Input: part model. Units: mm. Frame: model coordinates. Face numbers are marked on the shaded views. A direction names the side the tool comes from. Give positions to 0.01 mm unless a question says otherwise; leave off trailing zeros. Loops run counter-clockwise (first coordinate to the right, second up) from the corner with the lowest first, then second, coordinate; pieces in that order, holes last. Notation, with made-up numbers: (56.5, 53.25) -> (97.5, 53.25) arc R22 cw to (97.5, 85.25) -> close; hole circle Ø3 at (49.5, -38). An arc over 180 degrees is marked (long way). Answer in a Markdown table with one row per item. Add a question column.
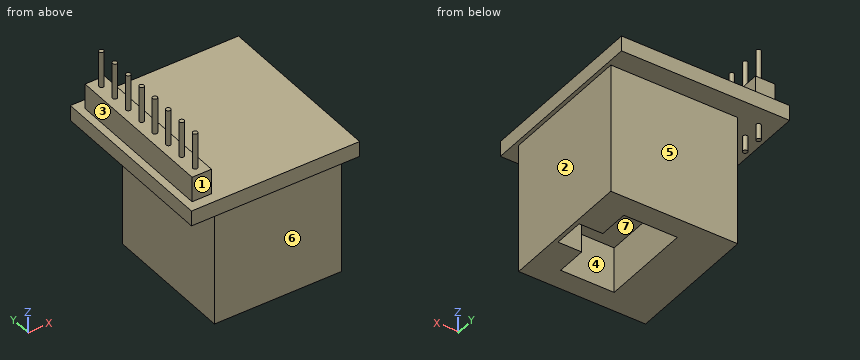
```python
from build123d import *

# Parameters (mm, degrees)
F0_W          = 16.6
F0_H          = 17.5
F1_DEPTH      = 17
F3_DEPTH      = 6
F4_W          = 22
F4_H          = 23
F4_W_2        = 16.6
F4_H_2        = 17.5
F5_DEPTH      = 2
F6_W          = 2.54
F6_H          = 2.54
F6_R          = 0.3
F7_DEPTH      = 3.3
F8_DEPTH      = 8
F8_DEPTH_BACK = 4


with BuildPart() as f1:
    # F0 (on Top) → F1 (new body)
    with BuildSketch(Plane.XY):
        Rectangle(F0_W, F0_H)
    extrude(amount=F1_DEPTH)

    # F2 (on face) → F3 (cut)
    with BuildSketch(Plane(origin=(0, 0, 0), x_dir=(1, 0, 0), z_dir=(0, 0, -1))):
        Polygon((7.8, -2), (7.8, 0), (7.8, 2), (4.7, 2), (4.7, 6), (-2.3, 6), (-2.3, 0), (-2.3, -6), (4.7, -6), (4.7, -2), align=None)
    extrude(amount=-F3_DEPTH, mode=Mode.SUBTRACT)

    # F4 (on face) → F5 (join)
    with BuildSketch(Plane.XY.offset(17)):
        with Locations((-2.2, 0)):
            Rectangle(F4_W, F4_H)
        Rectangle(F4_W_2, F4_H_2, mode=Mode.SUBTRACT)
        Rectangle(F4_W_2, F4_H_2)
    extrude(amount=F5_DEPTH)

    # F6 (on face) → F7 (join)
    with BuildSketch(Plane.XY.offset(19)):
        with Locations((-10.93, -8.89)):
            Rectangle(F6_W, F6_H)
        with Locations((-10.93, -8.89)):
            Circle(F6_R, mode=Mode.SUBTRACT)
        with Locations((-10.93, -6.35)):
            Rectangle(F6_W, F6_H)
        with Locations((-10.93, -6.35)):
            Circle(F6_R, mode=Mode.SUBTRACT)
        with Locations((-10.93, -3.81)):
            Rectangle(F6_W, F6_H)
        with Locations((-10.93, -3.81)):
            Circle(F6_R, mode=Mode.SUBTRACT)
        with Locations((-10.93, -1.27)):
            Rectangle(F6_W, F6_H)
        with Locations((-10.93, -1.27)):
            Circle(F6_R, mode=Mode.SUBTRACT)
        with Locations((-10.93, 1.27)):
            Rectangle(F6_W, F6_H)
        with Locations((-10.93, 1.27)):
            Circle(F6_R, mode=Mode.SUBTRACT)
        with Locations((-10.93, 8.89)):
            Rectangle(F6_W, F6_H)
        with Locations((-10.93, 8.89)):
            Circle(F6_R, mode=Mode.SUBTRACT)
        with Locations((-10.93, 3.81)):
            Rectangle(F6_W, F6_H)
        with Locations((-10.93, 3.81)):
            Circle(F6_R, mode=Mode.SUBTRACT)
        with Locations((-10.93, 6.35)):
            Rectangle(F6_W, F6_H)
        with Locations((-10.93, 6.35)):
            Circle(F6_R, mode=Mode.SUBTRACT)
    extrude(amount=F7_DEPTH)

    # F6 (on face) → F8 (join, two sides)
    with BuildSketch(Plane.XY.offset(19)) as f8_sk:
        with Locations((-10.93, -8.89)):
            Circle(F6_R)
        with Locations((-10.93, -6.35)):
            Circle(F6_R)
        with Locations((-10.93, -3.81)):
            Circle(F6_R)
        with Locations((-10.93, -1.27)):
            Circle(F6_R)
        with Locations((-10.93, 1.27)):
            Circle(F6_R)
        with Locations((-10.93, 3.81)):
            Circle(F6_R)
        with Locations((-10.93, 6.35)):
            Circle(F6_R)
        with Locations((-10.93, 8.89)):
            Circle(F6_R)
    extrude(amount=F8_DEPTH)
    extrude(f8_sk.sketch, amount=-F8_DEPTH_BACK)


solid = f1.part
```
1) Section C-C on y = 7.5. Output: boundary loops of the cut face in (x, z), and give its area (3 significant figures).
2) Reachability of the marked faces 1, 2, 3 and 4 from +Z, -Z, +X, -X, +Y, -Y: full face, straight path, thin tool, end or side. Return the list, or none.
3) Section A-A on z = 3.25. Output: boundary loops of the cut face in (x, y), and give its area (3 significant figures).
4) Pin query (flat end, axial travel): pin 1 (3 mm diameter, centred on y = -4, z = 3, fed in from -X); pin 2 (2.5 mm diameter, centred on y = 0, z = 21, fed in from +X); pin 3 (8.5 mm diameter, centred on y = -0.5, z = 10, fed in from +X). Return the tip coordinate at first contact, or that it passes through.
5) Section B-B on x = 7.25. Output: boundary loops of the cut face in (y, z), and give its area (4 significant figures).
6) Material intervals for line 1 along Y through (x, z) = (4.5, 2.25); line 2 along Z through (x, y) = (-3.25, -8); line 3 along X through (y, z) = (7.75, 15), sorted ascending.
7) Section D-D on z = 25.5. Output: boundary loops of the cut face in (x, y).
8) Pull-direction query (Y, two-part tool) for the marked faces 5, 6 and 7; classes: +Y half, -Y half, draft (parallel to the pull), parting line (faces both ways), or undercut.
Working result:
| question | item | result |
|---|---|---|
| 1 | outline | (-13.2, 17) -> (-8.3, 17) -> (-8.3, 0) -> (8.3, 0) -> (8.3, 17) -> (8.8, 17) -> (8.8, 19) -> (-9.66, 19) -> (-9.66, 22.3) -> (-12.2, 22.3) -> (-12.2, 19) -> (-13.2, 19) -> close |
| 1 | area | 335 mm2 |
| 2 | face 1 | +Z, +X, -X, -Y |
| 2 | face 2 | -Z, +X, +Y, -Y |
| 2 | face 3 | +Z, -X, +Y, -Y |
| 2 | face 4 | -Z |
| 3 | outline | (-8.3, -8.75) -> (8.3, -8.75) -> (8.3, 8.75) -> (-8.3, 8.75) -> close; hole (-2.3, -6) -> (4.7, -6) -> (4.7, -2) -> (7.8, -2) -> (7.8, 2) -> (4.7, 2) -> (4.7, 6) -> (-2.3, 6) -> close |
| 3 | area | 194 mm2 |
| 4 | pin 1 | stops at x = -8.3 |
| 4 | pin 2 | stops at x = -9.66 |
| 4 | pin 3 | stops at x = 8.3 |
| 5 | outline | (-11.5, 17) -> (-8.75, 17) -> (-8.75, 0) -> (-2, 0) -> (-2, 6) -> (2, 6) -> (2, 0) -> (8.75, 0) -> (8.75, 17) -> (11.5, 17) -> (11.5, 19) -> (-11.5, 19) -> close |
| 5 | area | 319.5 mm2 |
| 6 | line 1 | y = -8.75 to -6, 6 to 8.75 |
| 6 | line 2 | z = 0 to 19 |
| 6 | line 3 | x = -8.3 to 8.3 |
| 7 | outline | circle Ø0.6 at (-10.93, -8.89); circle Ø0.6 at (-10.93, -6.35); circle Ø0.6 at (-10.93, -3.81); circle Ø0.6 at (-10.93, -1.27); circle Ø0.6 at (-10.93, 1.27); circle Ø0.6 at (-10.93, 3.81); circle Ø0.6 at (-10.93, 6.35); circle Ø0.6 at (-10.93, 8.89) |
| 8 | face 5 | +Y half |
| 8 | face 6 | -Y half |
| 8 | face 7 | undercut |
